Design review of the part built by this model. Coordinates are the model's own, in mm. Coordinates: 2 decimals unless noted, no trailing zeros. Order: outer loops, then holes, each group sorted by start corner. A loop starts at its lowest first (then second) coordinate and runs counter-clockwise, first axis right, second up. Notation, with made-up numbers: (-14, 5) -> (8, 5) arc R17 cw to (8, 20) -> close; hole circle Ø1 at (-13, 64.5). An arc over 180 degrees is marked (long way). Use a Markdown table: item, result. Add a question column.
Q1. Add section B-B (z = 6). State the section outline as (x, y) points.
Q2. Wall thickness on probe 1 along X at (y, z) = (-0.5, 0); probe 2 along Z at (x, y) = (0, 0); probe 3 along X at (y, z) = (0.6, -4.5): over which ranges is each line inside the solid? List them lowest first.
Q3. Add section C-C (y = -0.5). State the section outline as (x, z) points, then the cut area to 3 significant figures.
Q4. Add section A-A (x = 0). State the section outline as (y, z) points.
Q5. The part is to be moulded in two halves that separate along Z. For faces 1 (the face through (100.17, -0.01, -23.9)), 2 (the face through (-1, 1, 11)), 3 (the face through (-9.76, -0.01, -2.17)), 4 (the face through (100.17, 0.01, 23.9)), say which applies: pulls with the +Z half, pulls with the -Z half, needs draft (parallel to the pull), parting line crosses it, or undercut.
from build123d import *

# Parameters (mm, degrees)
SKETCH2_W               = 203.2
SKETCH2_H               = 50.8
BOSS_EXTRUDE1_DEPTH     = 1
FILLET1_R               = 5
CUT_EXTRUDE1_DEPTH      = 105.731657105
CUT_EXTRUDE1_DEPTH_BACK = 105.731657105
SKETCH3_R               = 10


with BuildPart() as part:
    # Sketch2 → Boss-Extrude1 (new, symmetric)
    with BuildSketch(Plane(origin=(0, 0, 0), x_dir=(1, 0, 0), z_dir=(0, 1, 0))):
        Rectangle(SKETCH2_W, SKETCH2_H)
    extrude(amount=BOSS_EXTRUDE1_DEPTH, both=True)

    # Fillet1
    fillet1_edges = [part.edges().sort_by_distance(p)[0] for p in [
        (101.6, 0, 25.4),
        (-101.6, 0, 25.4),
        (-101.6, 0, -25.4),
        (101.6, 0, -25.4),
    ]]
    fillet(fillet1_edges, radius=FILLET1_R)

    # Sketch3 → Cut-Extrude1 (cut, two sides: drawn at the far end of the back side and taken through both)
    with BuildSketch(Plane(origin=(0, 0, 0), x_dir=(1, 0, 0), z_dir=(0, 1, 0)).offset(-CUT_EXTRUDE1_DEPTH_BACK)):
        with Locations(Location((0, 0, 0), (0, 0, 270))):
            Circle(SKETCH3_R)
    extrude(amount=CUT_EXTRUDE1_DEPTH + CUT_EXTRUDE1_DEPTH_BACK, mode=Mode.SUBTRACT)


solid = part.part
Established:
| question | item | result |
|---|---|---|
| 1 | outline | (-101.6, -1) -> (-8, -1) -> (-8, 1) -> (-101.6, 1) -> close; (8, -1) -> (101.6, -1) -> (101.6, 1) -> (8, 1) -> close |
| 2 | probe 1 | -101.6 to -10, 10 to 101.6 |
| 2 | probe 2 | -25.4 to -10, 10 to 25.4 |
| 2 | probe 3 | -101.6 to -8.93, 8.93 to 101.6 |
| 3 | outline | (-101.6, -20.4) arc R5 ccw to (-96.6, -25.4) -> (96.6, -25.4) arc R5 ccw to (101.6, -20.4) -> (101.6, 20.4) arc R5 ccw to (96.6, 25.4) -> (-96.6, 25.4) arc R5 ccw to (-101.6, 20.4) -> close; hole circle Ø20 at (0, 0) |
| 3 | area | 9,990 mm^2 |
| 4 | outline | (-1, -25.4) -> (1, -25.4) -> (1, -10) -> (-1, -10) -> close; (-1, 10) -> (1, 10) -> (1, 25.4) -> (-1, 25.4) -> close |
| 5 | face 1 | pulls with the -Z half |
| 5 | face 2 | needs draft |
| 5 | face 3 | undercut |
| 5 | face 4 | pulls with the +Z half |
